The model under review builds one solid part; all positions refer to its coordinate system, in mm. A direction names the side the tool comes from. Coordinates: 2 decimals unless noted, no trailing zeros. Loops run counter-clockwise (first coordinate to the right, second up) from the corner with the lowest first, then second, coordinate; pieces in that order, holes last. Notation, with made-up numbers: (8, 13) - (41, 13) arc R30 cw to (41, 47) - close; hole circle Ø8 at (63.25, -22). An arc over 180 degrees is marked (long way). One line per item, written item: value. Start each with the question number.
1. For faces 1 (the face through (-9.724, 7.395, -1.014)), 2 (the face through (9.74, 7.4, 0.99)), 3 (the face through (-9.74, 7.4, 0.99)), 4 (the face through (5, -11.6, 3)), 5 (the face through (6.26, 7.4, -0.99)), list the 3-axis set-ups (+Z, -Z, +X, -X, +Y, -Y) from which the entire face can be reached by the end or side of a thin tool; tool diameter is ignored.
2. Mouldability with a two-part tool opening along X and no side actions: class faces 6 (the face through (8, 15, 0)), 7 (the face through (0, 0, 0)), 8 (the face through (11, -4, 0)), 9 (the face through (-6.26, 7.4, -0.99)) as +X half, -X half, draft (parallel to the pull), parting line (faces both ways), or undercut.
3. Insertion check: P1, Ø3, axis at x = -8.5, z = -1.5, coming from the -Y side; P2, Ø4.5, axis at x = -3, z = 0.5, coming from the +Y side; P3, Ø1, axis at x = -8.5, z = 5, coming from the +Y side; P4, Ø2.5, axis at x = 8, y = 5, coming from the +Z side. Each pin has a flat end and moves straight along its axis. Give the tip position at first contact, or say it passes through.
4. To check wall thickness, follow line 1 (Y direction, x = -4, z = 5); line 2 (Z direction, x = 8.75, y = 11); line 3 (X direction, y = 6.75, z = 1). State the ranges of each line that lie inside material, in increasing order.
5. We need section C-C, the plane y = -5.5. Give the boundary of the cut face in (x, z) (3 decimals).
6. We need section A-A, the plane y = 5.25. Give the boundary of the cut face in (x, z), then the cut area to 3 significant figures.
7. We need section B-B, the plane x = 0. Give the boundary of the cut face in (y, z) (3 decimals).
from build123d import *

# Parameters (mm, degrees)
SKETCH1_R           = 7.875
BOSS_EXTRUDE1_DEPTH = 11.6
BOSS_EXTRUDE2_DEPTH = 8
BOSS_EXTRUDE3_DEPTH = 15
CHAMFER1_SIZE       = 1


with BuildPart() as part:
    # Sketch1 → Boss-Extrude1 (new body)
    with BuildSketch(Plane(origin=(0, 0, 0), x_dir=(1, 0, 0), z_dir=(0, 1, 0))):
        with Locations(Location((0, 0, 0), (0, 0, 270))):
            Circle(SKETCH1_R)
    extrude(amount=-BOSS_EXTRUDE1_DEPTH)

    # Sketch2 → Boss-Extrude2 (add)
    with BuildSketch(Plane(origin=(0, 0, 0), x_dir=(1, 0, 0), z_dir=(0, 1, 0))):
        with BuildLine():
            Line((-8, 3), (-7.28118294, 3))
            ThreePointArc((-7.28118294, 3), (-7.875, 0), (-7.28118294, -3))
            Line((-7.28118294, -3), (-8, -3))
            ThreePointArc((-8, -3), (-11, 0), (-8, 3))
        make_face()
        with BuildLine():
            Line((8, -3), (7.28118294, -3))
            ThreePointArc((7.28118294, -3), (7.875, 0), (7.28118294, 3))
            Line((7.28118294, 3), (8, 3))
            ThreePointArc((8, 3), (11, 0), (8, -3))
        make_face()
    extrude(amount=-BOSS_EXTRUDE2_DEPTH)

    # Sketch3 → Boss-Extrude3 (add)
    with BuildSketch(Plane(origin=(0, 0, 0), x_dir=(1, 0, 0), z_dir=(0, 1, 0))):
        Polygon((6.845299462, -2), (5.690598923, 0), (6.845299462, 2), (9.154700538, 2), (10.309401077, 0), (9.154700538, -2), align=None)
        Polygon((-5.690598923, 0), (-6.845299462, 2), (-9.154700538, 2), (-10.309401077, 0), (-9.154700538, -2), (-6.845299462, -2), align=None)
    extrude(amount=BOSS_EXTRUDE3_DEPTH)

    # Sketch4 → Revolve1 (revolve)
    with BuildSketch(Plane.XY, mode=Mode.PRIVATE) as revolve1_sk:
        with BuildLine():
            Line((0, -11.6), (5.15, -11.6))
            ThreePointArc((5.15, -11.6), (3.085551004, -14.073334609), (0, -15))
            Line((0, -15), (0, -11.6))
        make_face()
    revolve(revolve1_sk.sketch.rotate(Axis((0, -15, 0), (0, 1, 0)), 180), axis=Axis((0, -15, 0), (0, 1, 0)))

    # Chamfer1
    chamfer1_edges = [part.edges().sort_by_distance(p)[0] for p in [
        (0, -11.6, -7.875),
    ]]
    chamfer(chamfer1_edges, length=CHAMFER1_SIZE)


solid = part.part
Findings below:
1. face 1: -Z, -X, +Y
1. face 2: +Z, +X, +Y
1. face 3: +Z, -X, +Y
1. face 4: -Y
1. face 5: -Z, +Y
2. face 6: draft
2. face 7: undercut
2. face 8: +X half
2. face 9: undercut
3. P1: y = -11.34
3. P2: y = 0
3. P3: through
3. P4: z = 2
4. line 1: -11.6 to 0
4. line 2: -2 to 2
4. line 3: -9.73 to -6.27, 6.27 to 9.73
5. outline: (-8, -3) - (-7.281, -3) arc R7.875 ccw to (7.281, -3) - (8, -3) arc R3 ccw to (8, 3) - (7.281, 3) arc R7.875 ccw to (-7.281, 3) - (-8, 3) arc R3 ccw to start
6. outline: (-10.31, 0) - (-9.15, -2) - (-6.85, -2) - (-5.69, 0) - (-6.85, 2) - (-9.15, 2) - close; (5.69, 0) - (6.85, -2) - (9.15, -2) - (10.31, 0) - (9.15, 2) - (6.85, 2) - close
6. area: 27.7 mm2
7. outline: (-11.6, -6.875) - (-10.6, -7.875) - (0, -7.875) - (0, 7.875) - (-10.6, 7.875) - (-11.6, 6.875) - (-11.6, 5.15) arc R5.6 ccw to (-11.6, -5.15) - close
